Design review of the part built by this model. Coordinates are the model's own, in mm. A direction names the side the tool comes from. Coordinates: 2 decimals unless noted, no trailing zeros. Write each loop counter-clockwise with the first axis right and the second up, starting at its lowest first coordinate (ties: lowest second). Pieces come first, ordered by that corner, then holes.
Q1. Insertion check: pin 1 (1 mm diameter, centred on x = 0.5, y = 0, fed in from -Z); pin 2 (2 mm diameter, centred on x = 2, z = 22.5, fed in from -Y). Each pin has a flat end and moves straight along its axis. Give the tip position at first contact, or say it passes through.
Q2. Take a section at B-B (z = 2). Give the boundary of the cut face in (x, y).
Q3. For probe 1 along Z at (x, y) = (-1.8, 0.45); probe 2 along Z at (x, y) = (1.55, 0); probe 3 along Y at (x, z) = (-1.95, 2), list the stretches that pass through material, from the lowest coordinate up.
Q4. Mouldability with a two-part tool opening along Z and no side actions: class faces 5 (the flat face through (0, -2, 32)), 6 (the cylindrical face through (-1.63, 0.38, 0.81)), 7 (the flat face through (-1.05, -0.03, 3.4)), 8 (the flat face through (0, 0, 36)) as pulls with the +Z half, pulls with the -Z half, needs draft (parallel to the pull), parting line crosses it, or undercut.
Q5. Machinability: for faces 1 (the flat face through (0, 0, 5.5)), 2 (the cylindrical face through (0, -2, 34)), 3 (the cylindrical face through (1.617, -0.67, 32.246)), 4 (the flat face through (-2, 0, 0)), which of the approach directions +Z, -Z, +X, -X, +Y, -Y give a long, thin tool a straight path to every point of the face, cutting with its end or side? Answer none if there is none.
Q6. Take a section at D-D (z = 6.5). Give the boundary of the cut face in (x, y).
Q7. Take a section at A-A (y = 0). State how many separate pieces and enclosed holes the cut face has, and give its area (3 significant figures).
```python
from build123d import *

# Parameters (mm, degrees)
SKETCH1_R               = 2.5
BOSS_EXTRUDE1_DEPTH     = 32
SKETCH2_R               = 1.75
BOSS_EXTRUDE2_DEPTH     = 0.5
SKETCH4_R               = 2
BOSS_EXTRUDE3_DEPTH     = 3.5
CHAMFER1_SIZE           = 0.25
CUT_EXTRUDE1_DEPTH      = 37.173194495
CUT_EXTRUDE1_DEPTH_BACK = 37.173194495
SKETCH5_R               = 1.25
CUT_EXTRUDE2_DEPTH      = 37.173194509
CUT_EXTRUDE2_DEPTH_BACK = 37.173194509
SKETCH6_W               = 2.1
SKETCH6_H               = 5.5


with BuildPart() as part:
    # Sketch1 → Boss-Extrude1 (new body)
    with BuildSketch(Plane.XY):
        Circle(SKETCH1_R)
    extrude(amount=BOSS_EXTRUDE1_DEPTH)

    # Sketch2 → Boss-Extrude2 (add)
    with BuildSketch(Plane.XY.offset(32)):
        Circle(SKETCH2_R)
    extrude(amount=BOSS_EXTRUDE2_DEPTH)

    # Sketch4 → Boss-Extrude3 (add)
    with BuildSketch(Plane.XY.offset(32.5)):
        Circle(SKETCH4_R)
    extrude(amount=BOSS_EXTRUDE3_DEPTH)

    # Chamfer1
    chamfer1_edges = [part.edges().sort_by_distance(p)[0] for p in [
        (-2, 0, 32.5),
        (-2, 0, 36),
        (-2.5, 0, 32),
    ]]
    chamfer(chamfer1_edges, length=CHAMFER1_SIZE - 0.0001)  # a hair under: the kernel refuses the full size

    # Sketch5 → Cut-Extrude1 (cut, two sides: drawn at the far end of the back side and taken through both)
    with BuildSketch(Plane(origin=(0, 0, 0), x_dir=(0, 0, -1), z_dir=(1, 0, 0)).offset(-CUT_EXTRUDE1_DEPTH_BACK)):
        with Locations((-2, 0)):
            Circle(SKETCH5_R)
    extrude(amount=CUT_EXTRUDE1_DEPTH + CUT_EXTRUDE1_DEPTH_BACK, mode=Mode.SUBTRACT)

    # Sketch6 → Cut-Extrude2 (cut, two sides: drawn at the far end of the back side and taken through both)
    with BuildSketch(Plane(origin=(0, 0, 0), x_dir=(1, 0, 0), z_dir=(0, 1, 0)).offset(-CUT_EXTRUDE2_DEPTH_BACK)):
        with Locations((0, -2.75)):
            Rectangle(SKETCH6_W, SKETCH6_H)
    extrude(amount=CUT_EXTRUDE2_DEPTH + CUT_EXTRUDE2_DEPTH_BACK, mode=Mode.SUBTRACT)


solid = part.part
```
Response:
1. pin 1: stops at z = 5.5
1. pin 2: stops at y = -2.29
2. outline: (-2.17, -1.25) arc R2.5 ccw to (-1.05, -2.27) - (-1.05, -1.25) - close; (-2.17, 1.25) - (-1.05, 1.25) - (-1.05, 2.27) arc R2.5 ccw to start; (1.05, -2.27) arc R2.5 ccw to (2.17, -1.25) - (1.05, -1.25) - close; (1.05, 1.25) - (2.17, 1.25) arc R2.5 ccw to (1.05, 2.27) - close
3. probe 1: z = 0 to 0.83, 3.17 to 32, 32.61 to 35.89
3. probe 2: z = 0 to 0.75, 3.25 to 36
3. probe 3: y = -1.56 to -1.25, 1.25 to 1.56
4. face 5: undercut
4. face 6: undercut
4. face 7: needs draft
4. face 8: pulls with the +Z half
5. face 1: -Z, +Y, -Y
5. face 2: +Z
5. face 3: none
5. face 4: -Z, +X, -X, +Y, -Y
6. outline: circle Ø5 at (0, 0)
7. separate pieces: 3
7. enclosed holes: 0
7. area: 157 mm2
